Can you work these out from the model? Positions are in its coordinate system, mm. A direction names the side the tool comes from. Round coordinates to 2 decimals unless told otherwise and drop trailing zeros. Order: outer loops, then holes, each group sorted by start corner. A loop starts at its lowest first (then second) coordinate and runs counter-clockwise, first axis right, second up.
Q1. If we section it at B-B (x = 15.5): Please give me the cut outline in (y, z), plus the area to 3 significant figures.
Q2. If we section it at D-D (z = -17.5): Please give me the cut outline in (x, y), plus the area to 3 significant figures.
Q3. For faces 1 (the face through (28.161, 6.084, -17.302)), 2 (the face through (6, 12, 0)), which set-ups out of +Z, -Z, +X, -X, +Y, -Y let a thin tool reach every point of the face, with its end or its side?
Q4. Will these pins go through, and if not, where does the flat tip stop? P1, Ø5, axis at x = -4, z = 4.5, coming from the +Y side; P2, Ø4, axis at y = 31, z = 4, coming from the +X side.
Q5. If we section it at A-A (z = -9.5): Please give me the cut outline in (x, y).
Q6. If I drill on line 1 (Y direction, x = -12, z = 8.5); line 2 (X direction, y = 17, z = 3); line 3 (X direction, y = 2.5, z = 13.5), over which ranges is the centre line in solid material (lowest first)?
Q7. If we section it at C-C (y = 34.5): Please give me the cut outline in (x, z).
from build123d import *

# Parameters (mm, degrees)
SKETCH1_W           = 66
SKETCH1_H           = 42
BOSS_EXTRUDE1_DEPTH = 12
SKETCH2_W           = 12
SKETCH2_H           = 42
BOSS_EXTRUDE2_DEPTH = 26.995042498
CUT_EXTRUDE1_DEPTH  = 12


with BuildPart() as part:
    # Sketch1 → Boss-Extrude1 (new body)
    with BuildSketch(Plane(origin=(0, 0, 0), x_dir=(1, 0, 0), z_dir=(0, 1, 0))):
        Rectangle(SKETCH1_W, SKETCH1_H)
    extrude(amount=BOSS_EXTRUDE1_DEPTH)

    # Sketch2 → Boss-Extrude2 (add)
    with BuildSketch(Plane(origin=(0, 12, 0), x_dir=(1, 0, 0), z_dir=(0, 1, 0))):
        with Locations((-27, 0)):
            Rectangle(SKETCH2_W, SKETCH2_H)
    extrude(amount=BOSS_EXTRUDE2_DEPTH)

    # Sketch12 → Cut-Extrude1 (cut)
    with BuildSketch(Plane(origin=(0, 12, 0), x_dir=(1, 0, 0), z_dir=(0, 1, 0))):
        Polygon((33, -12.935780303), (33, -21), (23.965356614, -21), align=None)
        Polygon((33, 13.5), (33, 21), (23.455136658, 21), align=None)
    extrude(amount=-CUT_EXTRUDE1_DEPTH, mode=Mode.SUBTRACT)


solid = part.part
Solution:
1. outline: (0, -21) - (12, -21) - (12, 21) - (0, 21) - close
1. area: 504 mm2
2. outline: (-33, 0) - (27.91, 0) - (27.91, 12) - (-21, 12) - (-21, 39) - (-33, 39) - close
2. area: 1,050 mm2
3. face 1: -Z, +X, +Y, -Y
3. face 2: +Z, -Z, +X, +Y
4. P1: stops at y = 12
4. P2: stops at x = -21
5. outline: (-33, 0) - (33, 0) - (33, 12) - (-21, 12) - (-21, 39) - (-33, 39) - close
6. line 1: y = 0 to 12
6. line 2: x = -33 to -21
6. line 3: x = -33 to 32.37
7. outline: (-33, -21) - (-21, -21) - (-21, 21) - (-33, 21) - close
